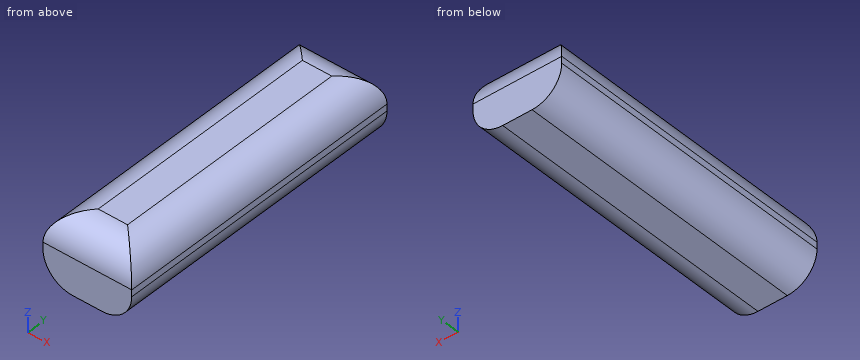
```python
from build123d import *

# Parameters (mm, degrees)
F0_W     = 75.895198
F0_H     = 56.5404
F1_DEPTH = 254
F2_R     = 25.4


with BuildPart() as f1:
    # F0 (on Front) → F1 (new body)
    with BuildSketch(Plane.XZ):
        with Locations((-37.947599, 28.2702)):
            Rectangle(F0_W, F0_H)
    extrude(amount=F1_DEPTH)

    # F2
    f2_edges = [f1.edges().sort_by_distance(p)[0] for p in [
        (0, -127, 56.5404),
        (0, -127, 0),
        (-75.895198, -127, 56.5404),
        (-37.947599, 0, 56.5404),
        (-37.947599, -254, 56.5404),
        (-75.895198, -127, 0),
    ]]
    fillet(f2_edges, radius=F2_R)


solid = f1.part
```
CAD build for the part. Positions are in the model's coordinates, mm. Coordinates: 2 decimals unless noted, no trailing zeros. Write each loop counter-clockwise with the first axis right and the second up, starting at its lowest first coordinate (ties: lowest second). Pieces come first, ordered by that corner, then holes. Notation, with made-up numbers: (78.5, 20) -> (90.5, 20) arc R21 ccw to (90.5, 45) -> close; hole circle Ø8 at (-26, 83.25). An arc over 180 degrees is marked (long way). Return JSON: item names as keys, results as strings. Group by question number.
Q1. Flat gauge pins, fed straight in: pin 1 (3 mm diameter, centred on x = -66.5, y = -170, fed in from +Z); pin 2 (12 mm diameter, centred on x = -12.5, y = -178.5, fed in from -Z); pin 3 (1 mm diameter, centred on x = -51.5, y = -77, fed in from -Z) (3 decimals). Where does each tip first touch, or does it go through?
Q2. Cut at C-C, the plane z = 12.5. Give the cut face in (x, y).
Q3. Cut at B-B, the plane x = -37. Give the cut face in (y, z), then the cut area to 3 significant figures.
Q4. Cut at D-D, the plane x = -15. Give the cut face in (y, z), then the cut area to 3 significant figures.
Q5. Drill centre lines: line 1 (X direction, y = -191, z = 25); line 2 (X direction, y = -32.5, z = 9); line 3 (Z direction, x = -69.5, y = -36). Where is each one in solid material? Low to high.
Q6. Cut at A-A, the plane y = -102. Give the cut face in (x, z), then the cut area to 3 significant figures.
Returned:
{
 "1": {"pin 1": "stops at z = 51.99", "pin 2": "stops at z = 0.96", "pin 3": "stops at z = 0.005"},
 "2": {"outline": "(-72.38, -254) -> (-3.52, -254) -> (-3.52, 0) -> (-72.38, 0) -> close"},
 "3": {"outline": "(-254, 0) -> (0, 0) -> (0, 31.14) arc R25.4 ccw to (-25.4, 56.54) -> (-228.6, 56.54) arc R25.4 ccw to (-254, 31.14) -> close", "area": "14,100 mm2"},
 "4": {"outline": "(-254, 2.23) -> (0, 2.23) -> (0, 31.14) arc R25.4 ccw to (-15, 54.31) -> (-239, 54.31) arc R25.4 ccw to (-254, 31.14) -> close", "area": "13,000 mm2"},
 "5": {"line 1": "x = -75.89 to 0", "line 2": "x = -69.89 to -6", "line 3": "z = 8.55 to 47.99"},
 "6": {"outline": "(-75.9, 25.4) arc R25.4 ccw to (-50.5, 0) -> (-25.4, 0) arc R25.4 ccw to (0, 25.4) -> (0, 31.14) arc R25.4 ccw to (-25.4, 56.54) -> (-50.5, 56.54) arc R25.4 ccw to (-75.9, 31.14) -> close", "area": "3,740 mm2"}
}
